CAD build for the part. Positions are in the model's coordinates, mm. A direction names the side the tool comes from. Coordinates: 2 decimals unless noted, no trailing zeros. Loops run counter-clockwise (first coordinate to the right, second up) from the corner with the lowest first, then second, coordinate; pieces in that order, holes last. Notation, with made-up numbers: (88.5, 20.5) -> (129.5, 20.5) arc R23 cw to (129.5, 44.5) -> close; hole circle Ø8 at (-16, -6). An arc over 180 degrees is marked (long way). Write each question's results on one line, items separated by ' | '.
```python
from build123d import *

# Parameters (mm, degrees)
SKETCH1_R           = 33
SKETCH1_R_2         = 3.65
BOSS_EXTRUDE1_DEPTH = 5


with BuildPart() as part:
    # Sketch1 → Boss-Extrude1 (new body)
    with BuildSketch(Plane.XY):
        Polygon((-85, 60), (-85, 65), (-75, 65), (-75, 60), (-45, 60), (-45, 65), (-35, 65), (-35, 60), (-5, 60), (-5, 65), (5, 65), (5, 60), (35, 60), (35, 65), (45, 65), (45, 60), (75, 60), (75, 65), (85, 65), (85, 60), (90, 60), (90, 35), (95, 35), (95, 25), (90, 25), (90, 5), (95, 5), (95, -5), (90, -5), (90, -25), (95, -25), (95, -35), (90, -35), (90, -60), (85, -60), (85, -65), (75, -65), (75, -60), (45, -60), (45, -65), (35, -65), (35, -60), (5, -60), (5, -65), (-5, -65), (-5, -60), (-35, -60), (-35, -65), (-45, -65), (-45, -60), (-75, -60), (-75, -65), (-85, -65), (-85, -60), (-90, -60), (-90, -35), (-95, -35), (-95, -25), (-90, -25), (-90, -5), (-95, -5), (-95, 5), (-90, 5), (-90, 25), (-95, 25), (-95, 35), (-90, 35), (-90, 60), align=None)
        with Locations((-30, 0)):
            Circle(SKETCH1_R, mode=Mode.SUBTRACT)
        with Locations((-30, -45)):
            Circle(SKETCH1_R_2, mode=Mode.SUBTRACT)
        with Locations((-30, 45)):
            Circle(SKETCH1_R_2, mode=Mode.SUBTRACT)
    extrude(amount=BOSS_EXTRUDE1_DEPTH)


solid = part.part
```
Q1. Cut at B-B on y = 0. Write the cut outline in (x, z), and give its area (3 significant figures).
Results are:
outline: (-95, 0) -> (-63, 0) -> (-63, 5) -> (-95, 5) -> close; (3, 0) -> (95, 0) -> (95, 5) -> (3, 5) -> close | area: 620 mm^2
Q2. Pull direction X, two halves, no side cores. Call faces 1 (the flat face through (-60, 60, 2)), 2 (the flat face through (-95, 0, 2)), 3 (the flat face through (-40, -65, 2)): +X half, -X half, draft (parallel to the pull), parting line (faces both ways), or undercut.
Results are:
face 1: undercut | face 2: -X half | face 3: draft
Q3. Drop flat-ended pins along their axis: pin 1 (1.5 mm diameter, centred on y = -18.5, z = 2.5, fed in from -X); pin 2 (2.5 mm diameter, centred on x = 93.5, z = 2, fed in from +Y); pin 3 (2.5 mm diameter, centred on x = 87.5, z = 2.5, fed in from -Y). Give the stop position or say it passes through.
Results are:
pin 1: x = -90 | pin 2: y = 35 | pin 3: y = -60
Q4. Cut at A-A on x = -30. Write the cut outline in (y, z), and give its area (3 significant figures).
Results are:
outline: (-60, 0) -> (-48.65, 0) -> (-48.65, 5) -> (-60, 5) -> close; (-41.35, 0) -> (-33, 0) -> (-33, 5) -> (-41.35, 5) -> close; (33, 0) -> (41.35, 0) -> (41.35, 5) -> (33, 5) -> close; (48.65, 0) -> (60, 0) -> (60, 5) -> (48.65, 5) -> close | area: 197 mm^2
Q5. Wall check: L1, parallel to Y at x = -30, z = 3.6; L2, parallel to X at y = -0.5, z = 0.35; L3, parallel to Y at x = -50.5, z = 2.75. Give the ranges that are in metal, low to high. Write a range as from..to.
Results are:
L1: -60..-48.65, -41.35..-33, 33..41.35, 48.65..60 | L2: -95..-63, 3..95 | L3: -60..-25.86, 25.86..60
Q6. Cut at D-D on z = 2.45. Give the number of separate pieces and of enclosed holes in the cut face, and give its area (3 significant figures).
Results are:
separate pieces: 1 | enclosed holes: 3 | area: 18,900 mm^2
Q7. Which spindle directions (+Z, -Z, +X, -X, +Y, -Y) get a long thin tool onto all of the face, cutting with end or side? Do faces 4 (the flat face through (-5, -63, 2)), 5 (the flat face through (45, 63, 2)), 6 (the flat face through (92, 35, 2)), 7 (the flat face through (88, -60, 2)), 8 (the flat face through (-85, -63, 2)). Say none if no direction does.
Results are:
face 4: +Z, -Z, -Y | face 5: +Z, -Z, +Y | face 6: +Z, -Z, +X, +Y | face 7: +Z, -Z, +X, -Y | face 8: +Z, -Z, -X, -Y
Q8. Cut at C-C on y = 45. Write the cut outline in (x, z).
Results are:
outline: (-90, 0) -> (-33.65, 0) -> (-33.65, 5) -> (-90, 5) -> close; (-26.35, 0) -> (90, 0) -> (90, 5) -> (-26.35, 5) -> close
